Check sheet for the modelled part. Datum: model origin and axes. Units: mm. Face numbers are marked on the shaded views. A direction names the side the tool comes from. Round coordinates to 2 decimals unless told otherwise and drop trailing zeros. Loops run counter-clockwise (first coordinate to the right, second up) from the corner with the lowest first, then second, coordinate; pieces in that order, holes last. Notation, with made-up numbers: (-32.75, -23.5) - (22.25, -23.5) arc R26 ccw to (22.25, -5.5) - close; hole circle Ø3 at (-21, -21). An arc over 180 degrees is marked (long way). Put each result on its own line as item: value. Start each with the question number.
Item 1: Gauge pin test, flat ends, axial feed: pin 1 Ø6 at (x, z) = (1.5, -10) entering from +Y; pin 2 Ø6 at (y, z) = (-0.5, -10.5) entering from -X; pin 3 Ø3.5 at (x, z) = (-1.5, -12) entering from -Y. Record the tip position at first contact, or that the pin passes through.
Item 2: Section check B-B, the plane x = 4.25. Record the cut outline in (y, z).
Item 3: Section check D-D, the plane y = 0. Give the number of separate pieces and of enclosed holes in the cut face, and give its area (3 significant figures).
Item 4: Material ranges on line 1 along Y through (x, z) = (-12, 2.3); line 2 along Z through (x, y) = (9.5, 1.5); line 3 along Z through (x, y) = (-4.75, 0.5), recorded low to high.
Item 5: Section check C-C, the plane z = -12.25. Record the cut outline in (x, y), and give its area (3 significant figures).
Item 6: Draft check along X on the marked faces 6, 7 and 8. Enter one of: pulls with the +X half, pulls with the -X half, needs draft (parallel to the pull), parting line crosses it, or undercut.
Item 7: Tool access check on the marked faces 1, 2, 3, 4 and 5. Record the directions out of +Z, -Z, +X, -X, +Y, -Y that give a thin tool (end or side, any length) a straight path to the whole face; none if there is none.
Item 8: Section check A-A, the plane x = -12. Record the cut outline in (y, z).
from build123d import *

# Parameters (mm, degrees)
SKETCH1_W           = 30
SKETCH1_H           = 10
SKETCH1_R           = 2
BOSS_EXTRUDE1_DEPTH = 5
SKETCH2_W           = 12
SKETCH2_H           = 8
BOSS_EXTRUDE2_DEPTH = 20
SKETCH3_R           = 5
CUT_EXTRUDE1_DEPTH  = 6


with BuildPart() as part:
    # Sketch1 → Boss-Extrude1 (new body)
    with BuildSketch(Plane.XY):
        Rectangle(SKETCH1_W, SKETCH1_H)
        with Locations((12, 0)):
            Circle(SKETCH1_R, mode=Mode.SUBTRACT)
        with Locations(Location((-12, 0, 0), (0, 0, 180))):
            Circle(SKETCH1_R, mode=Mode.SUBTRACT)
    extrude(amount=BOSS_EXTRUDE1_DEPTH)

    # Sketch2 → Boss-Extrude2 (add)
    with BuildSketch(Plane(origin=(0, 0, 0), x_dir=(-1, 0, 0), z_dir=(0, 0, -1))):
        Rectangle(SKETCH2_W, SKETCH2_H)
    extrude(amount=BOSS_EXTRUDE2_DEPTH)

    # Sketch3 → Cut-Extrude1 (cut)
    with BuildSketch(Plane(origin=(-5, -5, 0), x_dir=(-0.7071067811865477, 0.7071067811865475, 0), z_dir=(-0.7071067811865475, -0.7071067811865477, 0))):
        with Locations(Location((1.414213562, 10, 0), (0, 0, 180))):
            Circle(SKETCH3_R)
    extrude(amount=-CUT_EXTRUDE1_DEPTH, mode=Mode.SUBTRACT)


solid = part.part
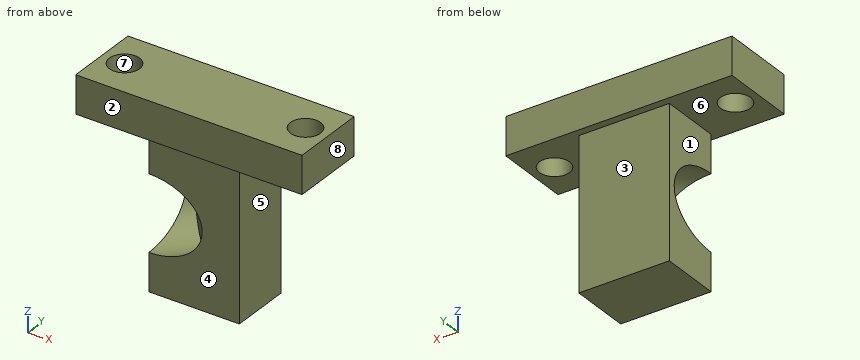
Check result:
1. pin 1: y = 4
1. pin 2: x = -4.01
1. pin 3: y = -4
2. outline: (-5, 0) - (-4, 0) - (-4, -20) - (4, -20) - (4, 0) - (5, 0) - (5, 5) - (-5, 5) - close
3. separate pieces: 3
3. enclosed holes: 0
3. area: 307 mm²
4. line 1: -5 to -2, 2 to 5
4. line 2: 0 to 5
4. line 3: -20 to -14.44, -5.56 to 5
5. outline: (-6, 2.31) - (-4.91, 3.4) - (1.4, -2.91) - (0.31, -4) - (6, -4) - (6, 4) - (-6, 4) - close
5. area: 62.4 mm²
6. face 6: needs draft
6. face 7: undercut
6. face 8: pulls with the +X half
7. face 1: -Z, -X, +Y, -Y
7. face 2: +Z, -Z, +X, -X, -Y
7. face 3: -Z, +X, -X, +Y
7. face 4: -Z, +X, -X, -Y
7. face 5: -Z, +X, +Y, -Y
8. outline: (-5, 0) - (-2, 0) - (-2, 5) - (-5, 5) - close; (2, 0) - (5, 0) - (5, 5) - (2, 5) - close
